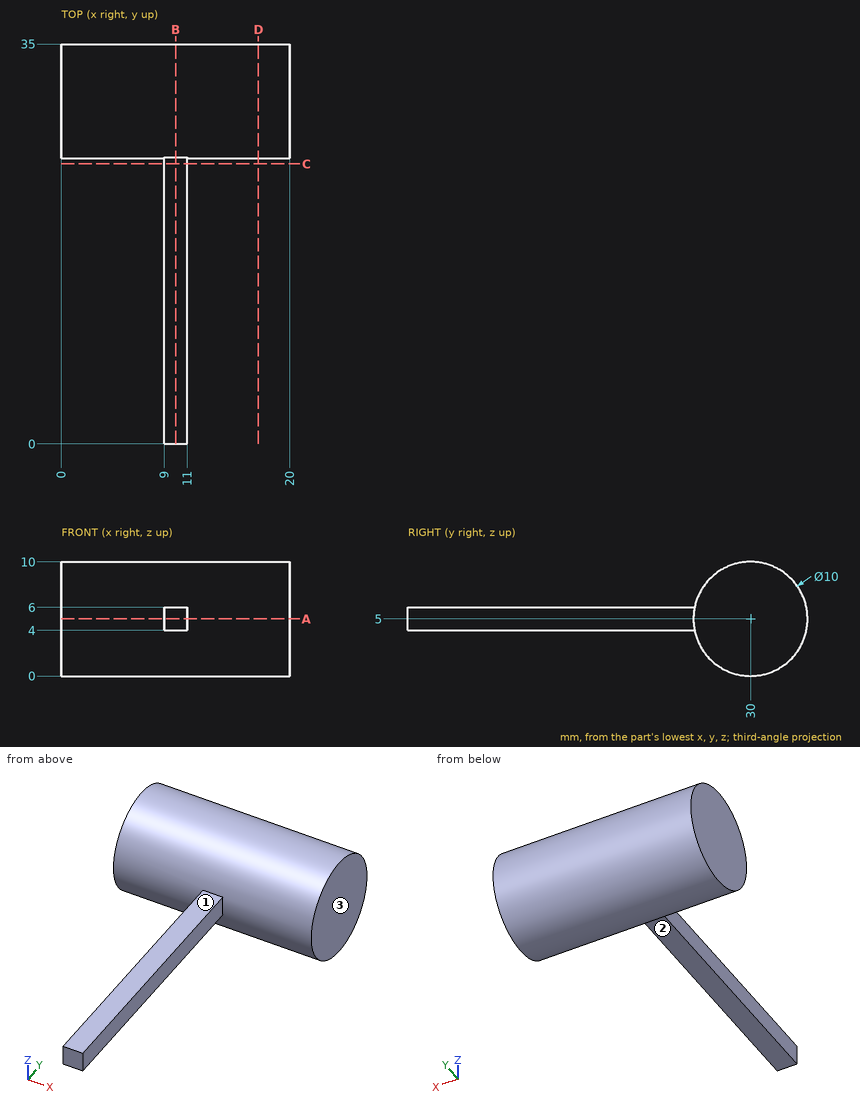
The figure shows three views and two pictorial views of one solid part (mm, origin at its lowest corner). Answer the questions. A direction names the side the tool comes from. Coordinates: 2 decimals unless noted, no trailing zeros. Loops run counter-clockwise (first coordinate to the right, second up) from the corner with the lowest first, then second, coordinate; pieces in that order, holes last.
(1) Consider line 1 along Y through (x, z) = (3, 5); line 2 along X through (y, z) = (23, 5.75); line 3 along Y through (x, z) = (6.5, 4). Determine where each line is inside the solid, lowest interval first.
Solution:
line 1: y = 25 to 35
line 2: x = 9 to 11
line 3: y = 25.1 to 34.9
(2) The part is cut by section B-B (x = 10). Determine the outline of the cut face in (y, z), and give its area (3 significant figures).
Solution:
outline: (0, 4) - (25.1, 4) arc R5 ccw (long way) to (25.1, 6) - (0, 6) - close
area: 129 mm2
(3) A tool of negligible diameter and unlimited length cuts with its end or side. For the marked faces 1, 2 and 3, from which of +Z, -Z, +X, -X, +Y, -Y can it reach the whole face along a straight path? Write none if from no direction.
Solution:
face 1: +Z, +X, -X, -Y
face 2: -Z, +X, -X, -Y
face 3: +Z, -Z, +X, +Y, -Y
(4) Flat-ended cylindrical pins translate along their axes: pin 1 Ø1.6 at (y, z) = (13.5, 5) entering from -X; pin 2 Ø1 at (x, y) = (12, 14.5) entering from +Z; pin 3 Ø10 at (x, y) = (5.5, 15.5) entering from -Z; pin 4 Ø1.5 at (y, z) = (23, 3.5) entering from +X. Find the tip coordinate at first contact, or state that the pin passes through.
Solution:
pin 1: stops at x = 9
pin 2: passes through
pin 3: stops at z = 4
pin 4: stops at x = 11
(5) The part is cut by section C-C (y = 24.5). Determine the outline of the cut face in (x, z), and give its area (3 significant figures).
Solution:
outline: (9, 4) - (11, 4) - (11, 6) - (9, 6) - close
area: 4.00 mm2
(6) The part is cut by section D-D (x = 17.25). Determine the outline of the cut face in (y, z).
Solution:
outline: circle Ø10 at (30, 5)
(7) The part is cut by section A-A (z = 5). Determine the outline of the cut face in (x, y), and give its area (3 significant figures).
Solution:
outline: (0, 25) - (9, 25) - (9, 0) - (11, 0) - (11, 25) - (20, 25) - (20, 35) - (0, 35) - close
area: 250 mm2
